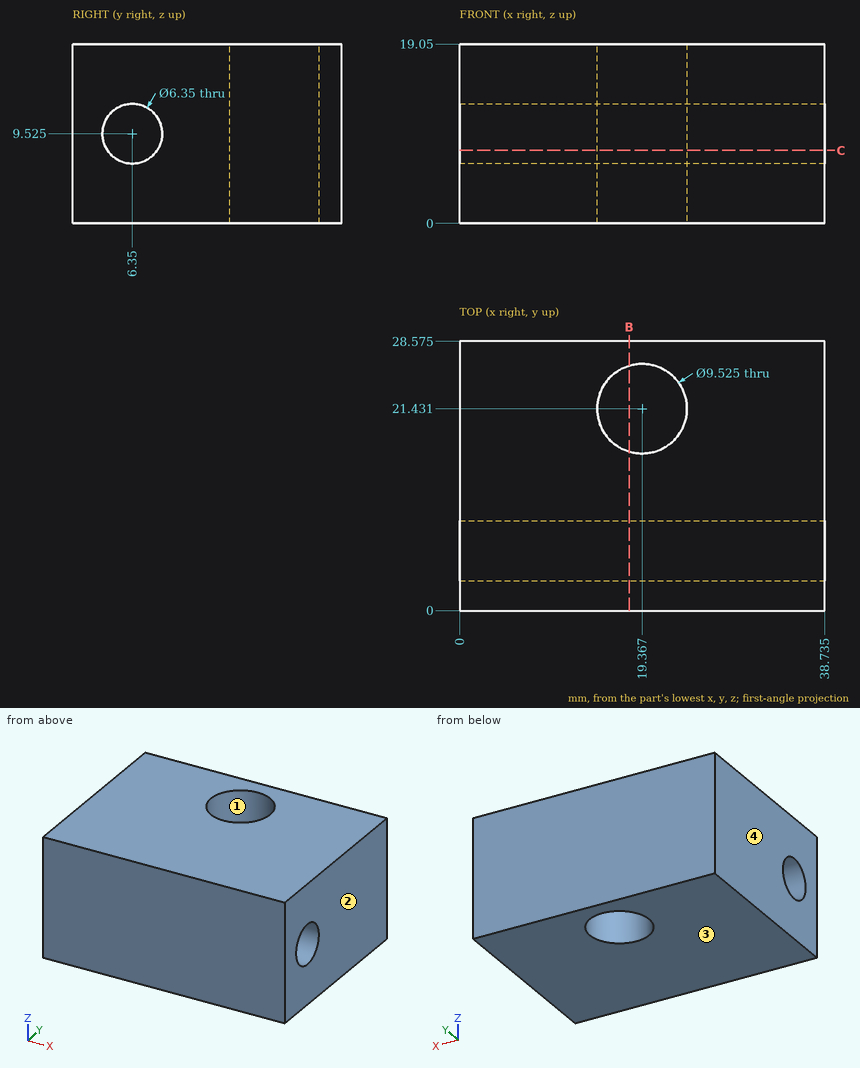
Input: dimensioned drawing with shaded views. Units: mm. Origin: part minimum x, y, z. Coordinates: 2 decimals unless noted, no trailing zeros. Order: outer loops, then holes, each group sorted by start corner. A loop starts at its lowest first (then second) coordinate and runs counter-clockwise, first axis right, second up.
(1) Section query B-B (x = 18). State how many separate pieces and enclosed holes the cut face has, plus the area to 3 significant figures.
(2) Draft query along X for the marked faces 1, 2, 3 and 4. Return one class per face: pulls with the +X half, pulls with the -X half, needs draft (parallel to the pull), parting line crosses it, or undercut.
(3) Section query C-C (z = 7.75). Return the cut outline in (x, y) (1 decimal).
(4) First-contact query: pin 1 (8.5 mm diameter, centred on x = 19.37, y = 21.43, fed in from -Z). Flat tip, straight axial feed; report the tip coordinate or a pass-through.
(5) Material intervals for probe 1 along X at (y, z) = (21.5, 7.5) (1 decimal); probe 2 along Z at (x, y) = (30.5, 6.5); probe 3 along Y at (x, z) = (34, 7.5) (1 decimal), sorted ascending.
Solution:
1. separate pieces: 2
1. enclosed holes: 1
1. area: 339 mm2
2. face 1: undercut
2. face 2: pulls with the +X half
2. face 3: needs draft
2. face 4: pulls with the -X half
3. outline: (0, 0) - (38.7, 0) - (38.7, 3.7) - (0, 3.7) - close; (0, 9) - (38.7, 9) - (38.7, 28.6) - (0, 28.6) - close; hole circle Ø9.5 at (19.4, 21.4)
4. pin 1: passes through
5. probe 1: x = 0 to 14.6, 24.1 to 38.7
5. probe 2: z = 0 to 6.35, 12.7 to 19.05
5. probe 3: y = 0 to 3.9, 8.8 to 28.6
